Autodesk Inventor part; units mm, degrees
ref_plane "YZ Plane" through (0, 0, 0) normal (1, 0, 0) x (0, 1, 0)
ref_plane "XZ Plane" through (0, 0, 0) normal (0, 1, 0) x (-1, 0, 0)
ref_plane "XY Plane" through (0, 0, 0) normal (0, 0, 1) x (1, 0, 0)
sketch "Sketch1" plane through (0, 0, 0) normal (0, 1, 0) x (-1, 0, 0)
  circle A0 centre (0, 0) radius 4
  dimension "d0" = 8
extrude "Extrusion1" add sketch "Sketch1" along normal blind 400
sketch "Sketch2" plane through (0, 400, 0) normal (0, 1, 0) x (1, 0, 0)
  circle A0 centre (0, 0) radius 4
  dimension "d3" = 8
extrude "Extrusion2" cut sketch "Sketch2" against normal blind 18
sketch "Sketch3" plane through (0, 382, 0) normal (0, 1, 0) x (1, 0, 0)
  circle A0 centre (0, 0) radius 4
  dimension "d6" = 8
extrude "Extrusion3" add sketch "Sketch3" along normal blind 100
properties part number "e_lead"
Design review of the part built by this model. Coordinates are the model's own, in mm. Round coordinates to 2 decimals unless told otherwise and drop trailing zeros. Loops run counter-clockwise (first coordinate to the right, second up) from the corner with the lowest first, then second, coordinate; pieces in that order, holes last. Notation, with made-up numbers: (44, -3) -> (88, -3) arc R20 cw to (88, 15) -> close; hole circle Ø2 at (55.25, -35). An arc over 180 degrees is marked (long way). Use one line per item in the form item = value. Start each with the question number.
Q1. We need section B-B on z = -2.5. Give the boundary of the cut face in (x, y).
Q2. We need section A-A on y = 421. Give the boundary of the cut face in (x, z), then the cut area to 3 significant figures.
Q3. Wall thickness on line 1 along X through (y, z) = (347, -0.25); line 2 along X through (y, z) = (370.5, 0.75); line 3 along Z through (x, y) = (0.5, 296): over which ranges is each line inside the solid? List them lowest first. Write a range as [from, to].
Q4. We need section C-C on x = 2.25. Give the boundary of the cut face in (y, z), then the cut area to 3 significant figures.
Q5. For pin 1 Ø1.5 at (x, z) = (-1.5, 1) entering from -Y; pin 2 Ø1.5 at (x, y) = (-2.5, 424) entering from +Z; pin 3 Ø4 at (x, y) = (3, 360.5) entering from +Z, all flat-tipped, find the tip position at first contact; note any pin that passes through.
Calculated:
q1.outline = (-3.12, 0) -> (3.12, 0) -> (3.12, 482) -> (-3.12, 482) -> close
q2.outline = circle Ø8 at (0, 0)
q2.area = 50.3 mm²
q3.line_1 = [-3.99, 3.99]
q3.line_2 = [-3.93, 3.93]
q3.line_3 = [-3.97, 3.97]
q4.outline = (0, -3.31) -> (482, -3.31) -> (482, 3.31) -> (0, 3.31) -> close
q4.area = 3,190 mm²
q5.pin_1 = 0
q5.pin_2 = 3.6
q5.pin_3 = 3.87
